Part model, mm, in its own coordinate system. A direction names the side the tool comes from. Round coordinates to 2 decimals unless told otherwise and drop trailing zeros. Loops run counter-clockwise (first coordinate to the right, second up) from the corner with the lowest first, then second, coordinate; pieces in that order, holes last. Notation, with made-up numbers: M -16.5,85.25 L 15.5,85.25 A21 cw 15.5,112.25 Z; hole C 68.25,50.5 d8. An arc over 180 degrees is marked long. Put each result on its own line as item: value. Start each with the question number.
1) Probe line 1 along Y through (x, z) = (150, 1.95); line 2 along Y through (x, z) = (734, 0.9); line 3 along X through (y, z) = (282, 0.35). List the from-to ranges inside material, lowest first.
2) Slice it at D-D on y = 280. Give the cut face in (x, z), then the cut area to 3 significant figures.
3) Slice it at B-B on y = 462.5. Give the cut face in (x, z), then the cut area to 3 significant figures.
4) Slice it at A-A on x = 730. Give the cut face in (y, z), then the cut area to 3 significant figures.
5) Pull direction Y, two halves, no side cores. Call faces 3 (the cylindrical face through (775.307, 594.268, 1.521)), 4 (the flat face through (513, 431, 3)): +Y half, -Y half, draft (parallel to the pull), parting line (faces both ways), or undercut.
6) Slice it at C-C on z = 1.65. Give the cut face in (x, y), then the cut area to 3 significant figures.
7) Which spindle directions (+Z, -Z, +X, -X, +Y, -Y) get a long thin tool onto all of the face, cutting with end or side? Do faces 1 (the cylindrical face through (440.66, 400.007, 1.521)), 2 (the flat face through (513, 431, 0)). Say none if no direction does.
```python
from build123d import *

# Parameters (mm, degrees)
SKETCH_1_W          = 850
SKETCH_1_H          = 850
EXTRUDE_1_DEPTH     = 3
SKETCH_2_R          = 47.5
CUT_EXTRUDE_1_DEPTH = 1203.085271518


with BuildPart() as part:
    # 草图1 → 凸台-拉伸1 (new body)
    with BuildSketch(Plane.XY):
        with Locations((425, 425)):
            Rectangle(SKETCH_1_W, SKETCH_1_H)
    extrude(amount=EXTRUDE_1_DEPTH)

    # 草图2 → 切除-拉伸1 (cut, through all)
    with BuildSketch(Plane.XY.offset(3)):
        with Locations((150, 580)):
            Circle(SKETCH_2_R)
        with Locations((150, 280)):
            Circle(SKETCH_2_R)
        with Locations((730, 280)):
            Circle(SKETCH_2_R)
        with Locations((730, 580)):
            Circle(SKETCH_2_R)
        with BuildLine():
            Line((470, 660), (470, 430))
            ThreePointArc((470, 430), (440, 400), (410, 430))
            Line((410, 430), (410, 660))
            ThreePointArc((410, 660), (440, 690), (470, 660))
        make_face()
    extrude(amount=-CUT_EXTRUDE_1_DEPTH, mode=Mode.SUBTRACT)


solid = part.part
```
Recorded:
1. line 1: y = 0 to 232.5, 327.5 to 532.5, 627.5 to 850
1. line 2: y = 0 to 232.67, 327.33 to 532.67, 627.33 to 850
1. line 3: x = 0 to 102.54, 197.46 to 682.54, 777.46 to 850
2. outline: M 0,0 L 102.5,0 L 102.5,3 L 0,3 Z; M 197.5,0 L 682.5,0 L 682.5,3 L 197.5,3 Z; M 777.5,0 L 850,0 L 850,3 L 777.5,3 Z
2. area: 1,980 mm2
3. outline: M 0,0 L 410,0 L 410,3 L 0,3 Z; M 470,0 L 850,0 L 850,3 L 470,3 Z
3. area: 2,370 mm2
4. outline: M 0,0 L 232.5,0 L 232.5,3 L 0,3 Z; M 327.5,0 L 532.5,0 L 532.5,3 L 327.5,3 Z; M 627.5,0 L 850,0 L 850,3 L 627.5,3 Z
4. area: 1,980 mm2
5. face 3: undercut
5. face 4: draft
6. outline: M 0,0 L 850,0 L 850,850 L 0,850 Z; hole C 150,280 d95; hole C 150,580 d95; hole M 410,430 A30 ccw 470,430 L 470,660 A30 ccw 410,660 Z; hole C 730,280 d95; hole C 730,580 d95
6. area: 678,000 mm2
7. face 1: +Z, -Z
7. face 2: -Z, +X, -X, +Y, -Y
